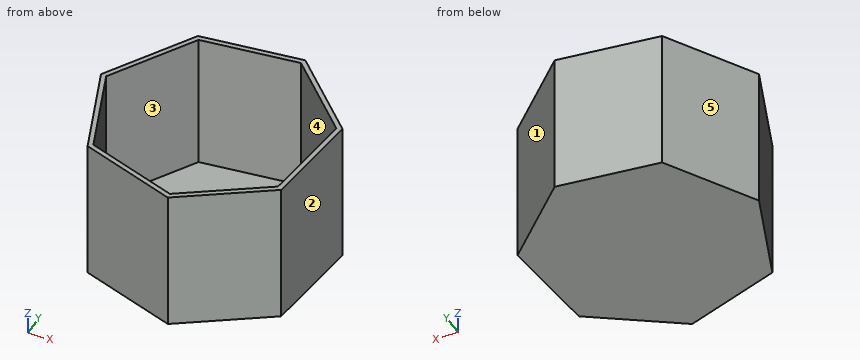
```python
from build123d import *

# Parameters (mm, degrees)
F1_DEPTH = 75.184
F2_T     = -101.6
F3_T     = -2.54


with BuildPart() as f1:
    # F0 (on Top) → F1 (new body)
    with BuildSketch(Plane.XY):
        Polygon((13.405336, 66.941666), (-38.520241, 59.935433), (-65.417615, 14.970067), (-47.032514, -34.094594), (2.790705, -50.311859), (46.534143, -21.469797), (51.258098, 30.712931), align=None)
    extrude(amount=F1_DEPTH)

    # F2
    f2_openings = [f1.faces().sort_by_distance(p)[0] for p in [
        (-5.283155, 9.526264, 75.184),
    ]]
    offset(amount=F2_T, openings=f2_openings)

    # F3
    f3_openings = [f1.faces().sort_by_distance(p)[0] for p in [
        (-5.283155, 9.526264, 75.184),
    ]]
    offset(amount=F3_T, openings=f3_openings)


solid = f1.part
```
The listing builds one solid part. Answer for the finished solid, in the listing's coordinates (mm). Face numbers are marked on the shaded views. A direction names the side the tool comes from. Give positions to 0.01 mm unless a question says otherwise; leave off trailing zeros. Write each loop counter-clockwise with the first axis right and the second up, starting at its lowest first coordinate (ties: lowest second). Pieces come first, ordered by that corner, then holes. Notation, with made-up numbers: (65, 7) - (86, 7) arc R23 cw to (86, 31) - close; hole circle Ø6 at (-2.5, 61.5). An arc over 180 degrees is marked (long way). Use one line per item in the form item = value. Start each with the question number.
1) Find section A-A on z = 65.5. Determine the outline of the cut face in (x, y), plus the area to 3 significant figures.
2) Consider line 1 along Z through (x, y) = (-7.5, -37.5); line 2 along Y through (x, z) = (15, 36); line 3 along X through (y, z) = (3, 71.5). Determine where each line is inside the solid, lowest interval first. Write a range as from..to.
3) Flat-ended cylindrical pins translate along their axes: pin 1 Ø8 at (x, z) = (17.5, 66) entering from -Y; pin 2 Ø1 at (x, y) = (26, -21.5) entering from +Z; pin 3 Ø3 at (x, z) = (-48.5, 66.5) entering from -Y. Find the tip coordinate at first contact, or state that the pin passes through.
4) Find section C-C on x = -5. Determine the outline of the cut face in (y, z), plus the area to 3 significant figures.
5) The mould has two halves that part along Y. Classify the marked faces 1, 2 and 3: pulls with the +Y half, pulls with the -Y half, needs draft (parallel to the pull), parting line crosses it, or undercut.
6) A tool of negligible diameter and unlimited length cuts with its end or side. For the marked faces 4 and 5, from which of +Z, -Z, +X, -X, +Y, -Y can it reach the whole face along a straight path? Write none if from no direction.
7) Find section B-B on y = -28.5. Determine the outline of the cut face in (x, z).
Geometry results:
q1.outline = (-65.42, 14.97) - (-47.03, -34.09) - (2.79, -50.31) - (46.53, -21.47) - (51.26, 30.71) - (13.41, 66.94) - (-38.52, 59.94) - close; hole (-62.61, 14.72) - (-45.08, -32.06) - (2.41, -47.52) - (44.11, -20.02) - (48.62, 29.72) - (12.53, 64.26) - (-36.97, 57.58) - close
q1.area = 910 mm2
q2.line_1 = 0..2.54
q2.line_2 = -42.26..-39.22, 61.9..65.42
q2.line_3 = -60.93..-58.22, 46.2..48.75
q3.pin_1 = -43.25
q3.pin_2 = 2.54
q3.pin_3 = -34.11
q4.outline = (-47.78, 0) - (64.46, 0) - (64.46, 75.18) - (61.9, 75.18) - (61.9, 2.54) - (-45.1, 2.54) - (-45.1, 75.18) - (-47.78, 75.18) - close
q4.area = 665 mm2
q5.face_1 = pulls with the +Y half
q5.face_2 = pulls with the -Y half
q5.face_3 = undercut
q6.face_4 = +Z
q6.face_5 = +Z, -Z, -X, +Y
q7.outline = (-49.13, 0) - (35.87, 0) - (35.87, 75.18) - (31.26, 75.18) - (31.26, 2.54) - (-46.42, 2.54) - (-46.42, 75.18) - (-49.13, 75.18) - close
